Source: CAD feature listing. Evaluate the final solid. Frame: model axes, mm. A direction names the side the tool comes from. Coordinates: 2 decimals unless noted, no trailing zeros. Loops run counter-clockwise (first coordinate to the right, second up) from the corner with the lowest first, then second, coordinate; pieces in that order, holes last. Notation, with made-up numbers: M -40,-7 L 14,-7 A22 cw 14,3 Z; hole C 27,29 d5. An arc over 180 degrees is marked long. One line per question, with ' | ' between items. Start each with the question number.
1. Section query A-A, the plane y = -9.75. Output: boundary loops of the cut face in (x, z), and give its area (3 significant figures).
2. Section query C-C, the plane x = -10. Output: boundary loops of the cut face in (y, z), and give its area (3 significant figures).
3. Ray query, probe 1 along X at (y, z) = (0, 21.75); probe 2 along X at (y, z) = (0, 26); probe 3 along Y at (x, z) = (0, 13.05). Return the intervals inside material, ascending.
4. Mould query, pull axis X, two halves, no side actions, for faces 3 (the cylindrical face through (-2.76, -8.764, 26.86)), 4 (the flat face through (12.3, -3.4, 27)), 5 (the cylindrical face through (-5.362, 12.932, 19.465)). Classes: pulls with the +X half, pulls with the -X half, needs draft (parallel to the pull), parting line crosses it, or undercut.
5. Access query for faces 1 (the cylindrical face through (0.66, -14.985, 24.465)), 2 (the cylindrical face through (-8.923, 1.172, 14.465)). Directions: +Z, -Z, +X, -X, +Y, -Y. A direction counts if a zero-diameter tool reaches every point of the face in a straight line with its end or side. Return the directions, or none.
6. Section query D-D, the plane z = 30. Output: boundary loops of the cut face in (x, y).
7. Pin query (flat end, axial travel): P1, Ø1.5, axis at x = 10.5, y = -11.5, coming from the -Z side; P2, Ø1, axis at x = 4, z = 4, coming from the +Y side; P3, Ø3, axis at y = 11.5, z = 17.5, coming from the -X side. Return the tip coordinate at first contact, or that it passes through.
8. Section query B-B, the plane z = 24. Output: boundary loops of the cut face in (x, y).
Autodesk Inventor part; units mm, degrees
ref_plane "YZ Plane" through (0, 0, 0) normal (1, 0, 0) x (0, 1, 0)
ref_plane "XZ Plane" through (0, 0, 0) normal (0, 1, 0) x (-1, 0, 0)
ref_plane "XY Plane" through (0, 0, 0) normal (0, 0, 1) x (1, 0, 0)
sketch "草圖1" plane through (0, 0, 0) normal (1, 0, 0) x (0, 1, 0)
  arc A0 (0, -5) -> (0, 5) centre (0, 0) ccw
  line L0 (0, 27) -> (12.5, 27)
  line L1 (12.5, 27) -> (12.5, 37)
  line L2 (12.5, 37) -> (0, 37)
  line L3 (0, 27) -> (15, 27)
  line L4 (15, 27) -> (15, 22)
  line L5 (15, 22) -> (0, 22)
  line L6 (0, 22) -> (0, 27)
  arc A1 (0, 3) -> (0, 31) centre (0, 17) ccw
  line L7 (14, 22) -> (14, 17)
  line L8 (0, 37) -> (0, -5)
  point P0 (3.5993, 3.4706)
  dimension "d0" = 10
  dimension "d2" = 12.5
  dimension "d3" = 10
  dimension "d4" = 15
  dimension "d10" = 20
  dimension "d11" = 5
  dimension "d12" = 27
revolve "迴轉1" add sketch "草圖1" angle 360 about axis through (0, 0, 37) along (0, 0, -1)
fillet "圓角1" radius 4 1 edges at (0, -3.5993, 3.4706)
sketch "草圖2" plane through (0, 0, 37) normal (0, 0, 1) x (1, 0, 0)
  point P0 (0, 0)
  point P1 (0, 0)
hole "孔1" at (0, 0, 37) direction (0, 0, -1) diameter 18 depth 25 tip angle 118
sketch "草圖3" plane through (0, 0, 37) normal (0, 0, 1) x (1, 0, 0)
  point P0 (0, 0)
  point P1 (0, 0)
hole "孔2" at (0, 0, 37) direction (0, 0, -1) diameter 18.376 depth 20
properties part number "3. 砲尾"
Taken from the geometry:
1) outline: M -11.4,22 L -10.05,22 L -10.05,17 A10.05 ccw 10.05,17 L 10.05,22 L 11.4,22 L 11.4,27 L 7.82,27 L 7.82,37 L -7.82,37 L -7.82,27 L -11.4,27 Z | area: 529 mm^2
2) outline: M -11.18,22 L -9.8,22 L -9.8,17 A9.8 ccw 9.8,17 L 9.8,22 L 11.18,22 L 11.18,27 L 7.5,27 L 7.5,37 L -7.5,37 L -7.5,27 L -11.18,27 Z | area: 511 mm^2
3) probe 1: -14 to -9.19, 9.19 to 14 | probe 2: -15 to -9.19, 9.19 to 15 | probe 3: -13.43 to -9, 9 to 13.43
4) face 3: undercut | face 4: needs draft | face 5: parting line crosses it
5) face 1: +Z, -Z | face 2: +Z
6) outline: C 0,0 d25; hole C 0,0 d18.38
7) P1: z = 22 | P2: y = 5.12 | P3: x = -9.8
8) outline: C 0,0 d30; hole C 0,0 d18.38
